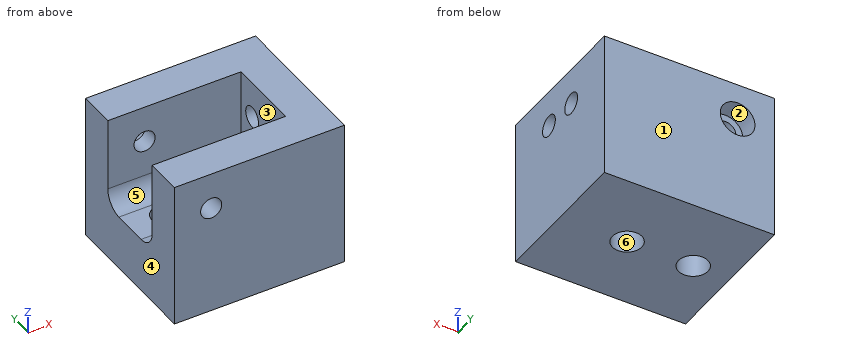
from build123d import *

# Parameters (mm, degrees)
SKETCH1_W                                      = 29.36875
SKETCH1_H                                      = 25.4
BOSS_EXTRUDE1_DEPTH                            = 25.4
SKETCH2_W                                      = 23.01875
SKETCH2_H                                      = 12.7
CUT_EXTRUDE1_DEPTH                             = 15.875
CBORE_FOR_6_SOCKET_HEAD_CAP_SCREW1_D           = 3.6576
CBORE_FOR_6_SOCKET_HEAD_CAP_SCREW1_CBORE_D     = 5.999999938
CBORE_FOR_6_SOCKET_HEAD_CAP_SCREW1_CBORE_DEPTH = 3.5052
F_6_CLEARANCE_HOLE2_D                          = 3.6576
FILLET1_R                                      = 3.175
TAP_DRILL_FOR_1_4_20_TAP2_D                    = 5.1054


with BuildPart() as part:
    # Sketch1 → Boss-Extrude1 (new body)
    with BuildSketch(Plane.XY):
        with Locations((14.684375, 12.7)):
            Rectangle(SKETCH1_W, SKETCH1_H)
    extrude(amount=BOSS_EXTRUDE1_DEPTH)

    # Sketch2 → Cut-Extrude1 (cut)
    with BuildSketch(Plane.XY.offset(25.4)):
        with Locations((11.509375, 12.7)):
            Rectangle(SKETCH2_W, SKETCH2_H)
    extrude(amount=-CUT_EXTRUDE1_DEPTH, mode=Mode.SUBTRACT)

    # CBORE for #6 Socket Head Cap Screw1 (through all)
    with Locations(Plane(origin=(0, 25.4, 0), x_dir=(1, 0, 0), z_dir=(0, 1, 0))):
        with Locations((6.35, -19.05)):
            CounterBoreHole(CBORE_FOR_6_SOCKET_HEAD_CAP_SCREW1_D / 2, CBORE_FOR_6_SOCKET_HEAD_CAP_SCREW1_CBORE_D / 2, CBORE_FOR_6_SOCKET_HEAD_CAP_SCREW1_CBORE_DEPTH)

    # #6 Clearance Hole2 (through all)
    with Locations(Plane(origin=(29.36875, 0, 0), x_dir=(0, 0, -1), z_dir=(1, 0, 0))):
        with Locations((-19.05, 15.875), (-19.05, 9.525)):
            Hole(F_6_CLEARANCE_HOLE2_D / 2)

    # Fillet1
    fillet1_edges = [part.edges().sort_by_distance(p)[0] for p in [
        (11.509375, 19.05, 9.525),
        (11.509375, 6.35, 9.525),
    ]]
    fillet(fillet1_edges, radius=FILLET1_R)

    # Tap Drill for 1/4-20 Tap2 (through all)
    with Locations(Plane.XY.offset(9.525)):
        with Locations((6.35, 12.7), (17.78, 12.7)):
            Hole(TAP_DRILL_FOR_1_4_20_TAP2_D / 2)


solid = part.part
Design review of the part built by this model. Coordinates are the model's own, in mm. Face numbers are marked on the shaded views. A direction names the side the tool comes from. Coordinates: 2 decimals unless noted, no trailing zeros. Loops run counter-clockwise (first coordinate to the right, second up) from the corner with the lowest first, then second, coordinate; pieces in that order, holes last. Notation, with made-up numbers: (69.5, 54.5) -> (126.5, 54.5) arc R29 ccw to (126.5, 86.5) -> close; hole circle Ø10 at (-28, 38.25). An arc over 180 degrees is marked (long way). Use a Markdown table: item, result. Add a question column.
Item 1: The part is to be moulded in two halves that separate along X. For the marked faces 4, 5 and 6, say which applies: +X half, -X half, draft (parallel to the pull), parting line (faces both ways), or undercut.
Item 2: We need section A-A, the plane y = 12.7. Write out the cut boundary in (x, z) (3 decimals).
Item 3: We need section D-D, the plane x = 6.35. Write out the cut boundary in (y, z) (3 decimals).
Item 4: We need section B-B, the plane x = 17.78. Write out the cut boundary in (y, z) (3 decimals).
Item 5: We need section C-C, the plane z = 19.05. Write out the cut boundary in (x, y), and give its area (3 significant figures).
Item 6: Wall thickness on L1, parallel to Y at x = 25, z = 19.05; L2, parallel to Y at x = 3, z = 13.5; L3, parallel to Y at x = 9.25, z = 18.5: over which ranges is each line inside the solid? List them lowest first. Write a range as from..to.
Item 7: Clearance check with flat-ended pins moving along their axes: P1, Ø4, axis at y = 15.5, z = 19, coming from the -X side; P2, Ø1.8, axis at x = 7, z = 18, coming from the +Y side; P3, Ø7, axis at x = 13.5, y = 12.5, coming from the +Z side. State where each tip first meets the part, or that it passes through.
Item 8: Machinability: for the marked faces 1, 2 and 3, which of the approach directions +Z, -Z, +X, -X, +Y, -Y give a long, thin tool a straight path to every point of the face, cutting with its end or side? Answer none if there is none.
Numbers:
| question | item | result |
|---|---|---|
| 1 | face 4 | -X half |
| 1 | face 5 | draft |
| 1 | face 6 | undercut |
| 2 | outline | (0, 0) -> (3.797, 0) -> (3.797, 9.525) -> (0, 9.525) -> close; (8.903, 0) -> (15.227, 0) -> (15.227, 9.525) -> (8.903, 9.525) -> close; (20.333, 0) -> (29.369, 0) -> (29.369, 25.4) -> (23.019, 25.4) -> (23.019, 9.525) -> (20.333, 9.525) -> close |
| 3 | outline | (0, 0) -> (10.147, 0) -> (10.147, 9.525) -> (9.525, 9.525) arc R3.175 cw to (6.35, 12.7) -> (6.35, 17.221) -> (0, 17.221) -> close; (0, 20.879) -> (6.35, 20.879) -> (6.35, 25.4) -> (0, 25.4) -> close; (15.253, 0) -> (25.4, 0) -> (25.4, 16.05) -> (21.895, 16.05) -> (21.895, 17.221) -> (19.05, 17.221) -> (19.05, 12.7) arc R3.175 cw to (15.875, 9.525) -> (15.253, 9.525) -> close; (19.05, 20.879) -> (21.895, 20.879) -> (21.895, 22.05) -> (25.4, 22.05) -> (25.4, 25.4) -> (19.05, 25.4) -> close |
| 4 | outline | (0, 0) -> (10.147, 0) -> (10.147, 9.525) -> (9.525, 9.525) arc R3.175 cw to (6.35, 12.7) -> (6.35, 25.4) -> (0, 25.4) -> close; (15.253, 0) -> (25.4, 0) -> (25.4, 25.4) -> (19.05, 25.4) -> (19.05, 12.7) arc R3.175 cw to (15.875, 9.525) -> (15.253, 9.525) -> close |
| 5 | outline | (0, 0) -> (4.52, 0) -> (4.52, 6.35) -> (0, 6.35) -> close; (0, 19.05) -> (4.52, 19.05) -> (4.52, 21.89) -> (3.35, 21.89) -> (3.35, 25.4) -> (0, 25.4) -> close; (8.18, 0) -> (29.37, 0) -> (29.37, 7.7) -> (23.02, 7.7) -> (23.02, 6.35) -> (8.18, 6.35) -> close; (8.18, 19.05) -> (23.02, 19.05) -> (23.02, 17.7) -> (29.37, 17.7) -> (29.37, 25.4) -> (9.35, 25.4) -> (9.35, 21.89) -> (8.18, 21.89) -> close; (23.02, 11.35) -> (29.37, 11.35) -> (29.37, 14.05) -> (23.02, 14.05) -> close |
| 5 | area | 353 mm^2 |
| 6 | L1 | y = 0..7.7, 11.35..14.05, 17.7..25.4 |
| 6 | L2 | y = 0..6.35, 19.05..25.4 |
| 6 | L3 | y = 0..6.35, 19.05..21.89 |
| 7 | P1 | stops at x = 23.02 |
| 7 | P2 | stops at y = 21.89 |
| 7 | P3 | stops at z = 9.57 |
| 8 | face 1 | +Z, -Z, +X, -X, +Y |
| 8 | face 2 | +Y |
| 8 | face 3 | +Z, -X |
